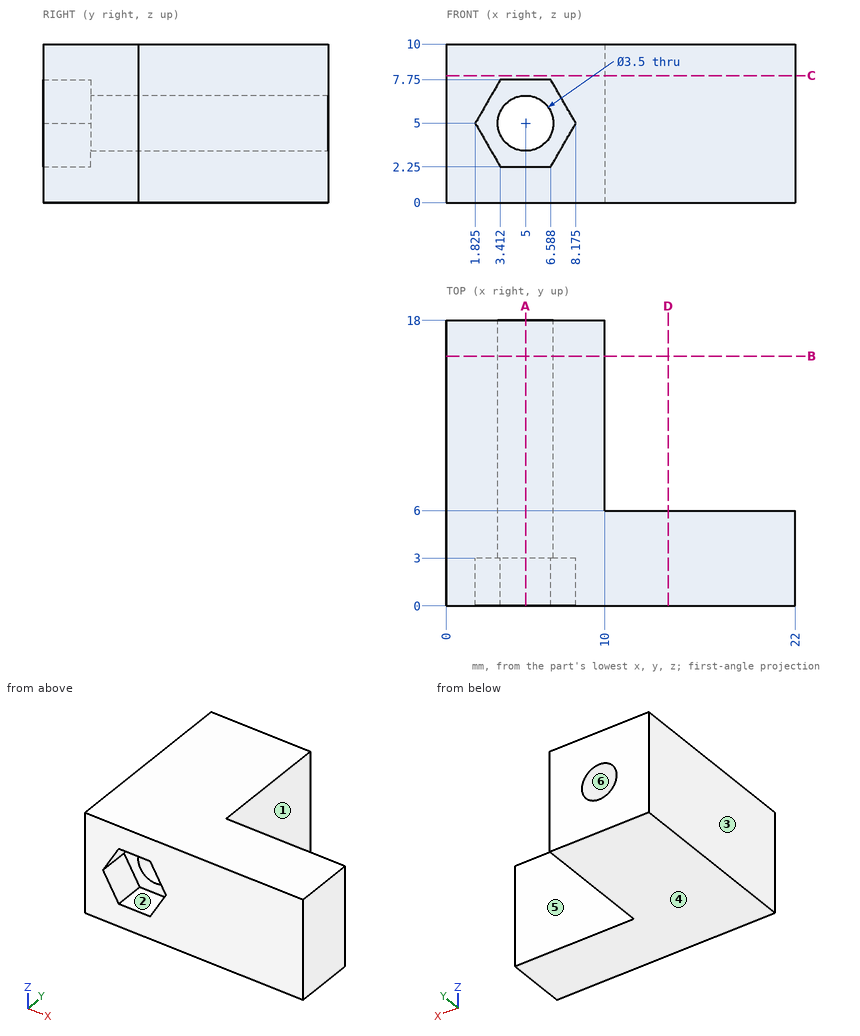
Study the drawing (mm; zero at the part's minimum x, y, z) and answer. A direction names the side the tool comes from. Give positions to 0.01 mm unless a question says otherwise; leave off trailing zeros. Loops run counter-clockwise (first coordinate to the right, second up) from the corner with the lowest first, then second, coordinate; pieces in that order, holes last. Notation, with made-up numbers: (68, -16.75) -> (72, -16.75) arc R21 cw to (72, 0.25) -> close; hole circle Ø9 at (42, 38). An arc over 180 degrees is marked (long way). Use a Markdown table: item, result. Add a question column.
1) Consider line 1 along X through (y, z) = (6.5, 5); line 2 along Z through (x, y) = (4.75, 2); line 3 along X through (y, z) = (16.5, 7). Determine where each line is inside the solid, lowest interval first.
2) The part is cut by section C-C, the plane z = 8. Determine the outline of the cut face in (x, y).
3) The part is cut by section B-B, the plane y = 15.75. Determine the outline of the cut face in (x, z).
4) Which of the six approach directions +Z, -Z, +X, -X, +Y, -Y give full straight-line access (tool end or side, diameter ignored) to the marked faces 1, 2 and 3?
5) For a pull along Z with two mould halves and no side action, classify the marked faces 4, 5 and 6 as +Z half, -Z half, draft (parallel to the pull), parting line (faces both ways), or undercut.
6) The part is cut by section D-D, the plane x = 14. Determine the outline of the cut face in (y, z), plus the area to 3 significant figures.
7) Each of these flat-tipped pins is pushed along its axis until it touches: P1, Ø1.5, axis at x = 11.5, z = 8, coming from the +Y side; P2, Ø3, axis at x = 5, z = 5, coming from the -Y side. Where does it stop, or does it pass through?
8) The part is cut by section A-A, the plane x = 5. Determine the outline of the cut face in (y, z).
Reported:
| question | item | result |
|---|---|---|
| 1 | line 1 | x = 0 to 3.25, 6.75 to 10 |
| 1 | line 2 | z = 0 to 2.25, 7.75 to 10 |
| 1 | line 3 | x = 0 to 10 |
| 2 | outline | (0, 0) -> (22, 0) -> (22, 6) -> (10, 6) -> (10, 18) -> (0, 18) -> close |
| 3 | outline | (0, 0) -> (10, 0) -> (10, 10) -> (0, 10) -> close; hole circle Ø3.5 at (5, 5) |
| 4 | face 1 | +Z, -Z, +X, +Y |
| 4 | face 2 | -Y |
| 4 | face 3 | +Z, -Z, -X, +Y, -Y |
| 5 | face 4 | -Z half |
| 5 | face 5 | draft |
| 5 | face 6 | undercut |
| 6 | outline | (0, 0) -> (6, 0) -> (6, 10) -> (0, 10) -> close |
| 6 | area | 60.0 mm^2 |
| 7 | P1 | stops at y = 6 |
| 7 | P2 | passes through |
| 8 | outline | (0, 0) -> (18, 0) -> (18, 3.25) -> (3, 3.25) -> (3, 2.25) -> (0, 2.25) -> close; (0, 7.75) -> (3, 7.75) -> (3, 6.75) -> (18, 6.75) -> (18, 10) -> (0, 10) -> close |
